Build history of the part. All positions in model axes, mm. Coordinates: 2 decimals unless noted, no trailing zeros. Order: outer loops, then holes, each group sorted by start corner. A loop starts at its lowest first (then second) coordinate and runs counter-clockwise, first axis right, second up. Notation, with made-up numbers: M 16.5,62 L 67.5,62 A21 ccw 67.5,96 Z; hole C 67,74 d10. An arc over 180 degrees is marked long. Use a Markdown table: item, result. Add a question column.
Autodesk Inventor part; units mm, degrees
ref_plane "YZ Plane" through (0, 0, 0) normal (1, 0, 0) x (0, 1, 0)
ref_plane "XZ Plane" through (0, 0, 0) normal (0, 1, 0) x (-1, 0, 0)
ref_plane "XY Plane" through (0, 0, 0) normal (0, 0, 1) x (1, 0, 0)
sketch "스케치1" plane through (0, 0, 0) normal (0, 1, 0) x (-1, 0, 0)
  line L0 (60, 80) -> (-60, 80)
  line L1 (-60, 80) -> (-60, -80)
  line L2 (-60, -80) -> (60, -80)
  line L3 (60, -80) -> (60, 80)
  line L4 (60, 80) -> (-60, -80) construction
  line L5 (-60, 80) -> (60, -80) construction
  point P0 (0, 0)
  dimension "d0" = 120
  dimension "d1" = 160
extrude "돌출1" add sketch "스케치1" along normal blind 60
sketch "스케치2" plane through (0, 60, 0) normal (0, 1, 0) x (1, 0, 0)
  line L0 (60, -80) -> (60, 80)
  line L1 (60, 80) -> (-60, 80)
  line L2 (55, 102.1646) -> (-55, 102.1646)
  line L3 (-55, 102.1646) -> (-55, -89.711)
  line L4 (-55, -89.711) -> (55, -89.711)
  line L5 (55, -89.711) -> (55, 102.1646)
  line L6 (-60, 80) -> (-60, -80)
  point P0 (0, 0)
  point P1 (55, 80)
  point P2 (-55, 80)
  dimension "d6" = 5
  dimension "d7" = 5
extrude "돌출2" cut sketch "스케치2" against normal blind 40 contours L5 L4 L3 L1
sketch "스케치12" plane through (60, 0, -80) normal (0, 0, -1) x (-1, 0, 0)
  line L0 (-34.8463, 10) -> (156.2634, 10)
  line L1 (156.2634, 10) -> (156.2634, -36.9465)
  line L2 (156.2634, -36.9465) -> (-34.8463, -36.9465)
  line L3 (-34.8463, -36.9465) -> (-34.8463, 10)
  line L4 (0, 0) -> (120, 0)
  point P0 (60, 0)
  dimension "d85" = 10
extrude "돌출10" cut sketch "스케치12" against normal through all
sketch "스케치13" plane through (-55, 20, 80) normal (0, 0, 1) x (1, 0, 0)
  line L0 (0, 40) -> (0, 0)
  line L1 (0, 0) -> (110, 0)
  line L2 (0, 40) -> (110, 40)
  line L3 (110, 40) -> (110, 0)
  line L4 (110, 0) -> (0, 0)
  line L5 (0, 0) -> (0, 40)
  point P0 (55, -20)
extrude "돌출11" add sketch "스케치13" against normal blind 5
sketch "스케치14" plane through (55, 20, -80) normal (0, 0, -1) x (-1, 0, 0)
  line L0 (0, 0) -> (0, 40)
  line L1 (110, 0) -> (0, 0)
  line L2 (0, 40) -> (110, 40)
  line L3 (110, 40) -> (110, 0)
  line L4 (110, 0) -> (0, 0)
  line L5 (0, 0) -> (0, 40)
  point P0 (55, -20)
extrude "돌출12" add sketch "스케치14" against normal blind 5
sketch "스케치15" plane through (60, 60, -80) normal (0, 0, -1) x (-1, 0, 0)
  point P0 (60, -60)
sketch "스케치16" plane through (60, 60, -80) normal (0, 0, -1) x (-1, 0, 0)
  point P0 (60, -60)
sketch "스케치17" plane through (0, 20, 0) normal (0, 1, 0) x (1, 0, 0)
  line L0 (7, 27) -> (45, 27)
  line L1 (45, 27) -> (45, 65)
  line L2 (45, 65) -> (7, 65)
  line L3 (7, 65) -> (7, 27)
  line L4 (55, 75) -> (55, -75)
  line L5 (55, 75) -> (-55, 75)
  circle A0 centre (7, 27) radius 1.6
  circle A1 centre (7, 65) radius 1.6
  circle A2 centre (45, 65) radius 1.6
  circle A3 centre (45, 27) radius 1.6
  line L6 (-47.9371, 14.7215) -> (-7.9371, 14.7215)
  line L7 (-7.9371, 14.7215) -> (-7.9371, 64.7215)
  line L8 (-7.9371, 64.7215) -> (-47.9371, 64.7215)
  line L9 (-47.9371, 64.7215) -> (-47.9371, 14.7215)
  point P0 (0, 0)
  dimension "d92" = 38
  dimension "d93" = 38
  dimension "d95" = 10
  dimension "d96" = 10
  dimension "d97" = 3.2
  dimension "d98" = 3.2
  dimension "d99" = 3.2
  dimension "d100" = 3.2
  dimension "d113" = 40
  dimension "d114" = 50
extrude "돌출13" cut sketch "스케치17" against normal through all contours L3 A0 L0 | L0 A0 L3 | A3 L1 L0 | L0 L1 A3 | A1 L2 L3 | L3 L2 A1 | A2 L2 L1 | L1 L2 A2
sketch "스케치21" plane through (0, 20, 0) normal (0, 1, 0) x (1, 0, 0)
  circle A0 centre (5.4243, 8.1678) radius 7.5
  line L0 (-49.3888, 17.2731) -> (-9.3888, 17.2731)
  line L1 (-9.3888, 17.2731) -> (-9.3888, 67.2731)
  line L2 (-9.3888, 67.2731) -> (-49.3888, 67.2731)
  line L3 (-49.3888, 67.2731) -> (-49.3888, 17.2731)
  point P0 (0, 0)
  dimension "d117" = 15
  dimension "d118" = 50
  dimension "d119" = 40
extrude "돌출15" cut sketch "스케치21" against normal through all contours A0
sketch "스케치23" plane through (0, 20, 0) normal (0, 1, 0) x (1, 0, 0)
  line L0 (-48.6, -65) -> (20, -65)
  line L1 (20, -65) -> (20, -11.6)
  line L2 (20, -11.6) -> (-48.6, -11.6)
  line L3 (-48.6, -11.6) -> (-48.6, -65)
  line L4 (55, 75) -> (55, -75)
  line L5 (-55, -75) -> (55, -75)
  circle A0 centre (4.7, -62.45) radius 1.6
  circle A1 centre (6.03, -14.15) radius 1.6
  circle A2 centre (-46.05, -47.16) radius 1.6
  circle A3 centre (-46.05, -19.23) radius 1.6
  point P0 (0, 0)
  dimension "d123" = 68.6
  dimension "d124" = 53.4
  dimension "d125" = 35
  dimension "d126" = 10
  dimension "d127" = 3.2
  dimension "d128" = 15.3
  dimension "d129" = 2.55
  dimension "d130" = 3.2
  dimension "d131" = 13.97
  dimension "d132" = 2.55
  dimension "d133" = 3.2
  dimension "d134" = 35.56
  dimension "d135" = 3.2
  dimension "d136" = 2.55
  dimension "d137" = 2.55
  dimension "d138" = 7.63
extrude "돌출16" cut sketch "스케치23" against normal through all contours A0 | A1 | A2 | A3
sketch "스케치24" plane through (0, 60, 0) normal (0, 1, 0) x (1, 0, 0)
  line L0 (-60, 80) -> (-60, -80)
  line L1 (60, 80) -> (-60, 80)
  line L2 (-60, -80) -> (60, -80)
  line L3 (60, -80) -> (60, 80)
  line L4 (60, 80) -> (-60, 80)
  line L5 (-60, 80) -> (-60, -80)
  point P0 (0, 0)
extrude "돌출17" cut sketch "스케치24" against normal blind 40
sketch "스케치25" plane through (60, 20, -80) normal (0, 0, -1) x (-1, 0, 0)
  point P0 (60, -20)
sketch "스케치26" plane through (0, 20, 0) normal (0, 1, 0) x (1, 0, 0)
  point P0 (0, 0)
sketch "스케치27" plane through (0, 20, 0) normal (0, 1, 0) x (1, 0, 0)
  line L0 (-60, -80) -> (-60, 80)
  line L1 (60, 80) -> (60, -80)
  line L2 (-60, -80) -> (60, -80)
  line L3 (60, -80) -> (60, 80)
  line L4 (60, 80) -> (-60, 80)
  line L5 (-60, 80) -> (-60, -80)
  point P0 (0, 0)
  point P1 (60, -80)
extrude "돌출18" cut sketch "스케치27" against normal blind 7
sketch "스케치28" plane through (0, 13, 0) normal (0, 1, 0) x (1, 0, 0)
  line L0 (-68.1907, -15.5) -> (-57, -15.5)
  line L1 (-57, -15.5) -> (-57, 15.5)
  line L2 (-57, 15.5) -> (-68.1907, 15.5)
  line L3 (-68.1907, 15.5) -> (-68.1907, -15.5)
  line L4 (-60, -80) -> (-60, 80)
  line L5 (60, -80) -> (-60, -80)
  line L6 (-15.5, -89.4714) -> (15.5, -89.4714)
  line L7 (15.5, -89.4714) -> (15.5, -77)
  line L8 (15.5, -77) -> (-15.5, -77)
  line L9 (-15.5, -77) -> (-15.5, -89.4714)
  line L10 (-60, 0) -> (60, 0)
  line L11 (0, 80) -> (0, -80)
  line L12 (-60, -80) -> (60, -80)
  line L13 (-15.5, 89.4714) -> (15.5, 89.4714)
  line L14 (15.5, 89.4714) -> (15.5, 77)
  line L15 (15.5, 77) -> (-15.5, 77)
  line L16 (-15.5, 77) -> (-15.5, 89.4714)
  line L17 (68.1907, -15.5) -> (57, -15.5)
  line L18 (57, -15.5) -> (57, 15.5)
  line L19 (57, 15.5) -> (68.1907, 15.5)
  line L20 (68.1907, 15.5) -> (68.1907, -15.5)
  point P0 (0, 0)
  dimension "d145" = 3
  dimension "d146" = 64.5
  dimension "d147" = 31
  dimension "d148" = 31
  dimension "d149" = 44.5
  dimension "d152" = 3
extrude "돌출19" cut sketch "스케치28" against normal through all contours L3 L2 L4 L0 | L15 L16 L13 L14 | L18 L19 L20 L17 | L4 L10 L1 L0 | L4 L2 L1 L10 | L9 L8 L11 L5 | L5 L7 L6 L9 | L11 L8 L7 L5
properties part number "본체 뚜껑 레이저"
(1) Mould opens along Z. For faces 1 (the cylindrical face through (-47.65, 11.52, 47.09)), 2 (the flat face through (1, 10, -1)) say: released by +Z, released by -Z, zero draft, split by the parting line, or undercut.
(2) Slice it at B-B on x = -12.5. Give the cut face in (y, z), and give its area (3 significant figures).
(3) Drop flat-ended pins along their axis: P1, Ø1.5, axis at x = 10, y = 10.5, coming from the -Z side; P2, Ø0.9, axis at y = 11, z = 6.5, coming from the +X side. Give the stop position or say it passes through.
(4) Slice it at A-A on y = 12.45. State how many separate pieces and enclosed holes the cut face has, and give its area (3 significant figures).
(5) Drill centre lines: line 1 along X through (y, z) = (10.2, -65); line 2 along X through (y, z) = (11.25, 19.23); line 3 along Z through (x, y) = (6.5, 12.15). Where is each one in solid material? Low to high. Write a range as from..to.
Solutions:
| question | item | result |
|---|---|---|
| 1 | face 1 | undercut |
| 1 | face 2 | zero draft |
| 2 | outline | M 10,-77 L 13,-77 L 13,77 L 10,77 Z |
| 2 | area | 462 mm² |
| 3 | P1 | z = -77 |
| 3 | P2 | x = 57 |
| 4 | separate pieces | 1 |
| 4 | enclosed holes | 9 |
| 4 | area | 18,600 mm² |
| 5 | line 1 | -60..5.4, 8.6..43.4, 46.6..60 |
| 5 | line 2 | -60..-47.65, -44.45..60 |
| 5 | line 3 | -77..-66.52, -63.48..-28.52, -25.48..-15.59, -0.75..12.62, 15.68..77 |
